Autodesk Inventor part; units mm, degrees
ref_plane "YZ Plane" through (0, 0, 0) normal (1, 0, 0) x (0, 1, 0)
ref_plane "XZ Plane" through (0, 0, 0) normal (0, 1, 0) x (-1, 0, 0)
ref_plane "XY Plane" through (0, 0, 0) normal (0, 0, 1) x (1, 0, 0)
sketch "Sketch1" plane through (0, 0, 0) normal (1, 0, 0) x (0, 1, 0)
  circle A0 centre (0, 0) radius 136.5
  dimension "d0" = 273
extrude "Extrude1" add sketch "Sketch1" along normal blind 432
sketch "Sketch2" plane through (0, 0, 0) normal (0, 0, 1) x (1, 0, 0)
  line L0 (0, 136.5) -> (0, -136.5)
  line L1 (432, 136.5) -> (432, -136.5)
  line L2 (0, 0) -> (432, 0) construction
  circle A0 centre (216, 0) radius 57.15
  dimension "d3" = 114.3
extrude "Extrude2" add sketch "Sketch2" along normal blind 184
sketch "Sketch3" plane through (0, 0, 0) normal (-1, 0, 0) x (0, 0, 1)
  circle A0 centre (0, 0) radius 136.5
  circle A1 centre (0, 0) radius 130.2
  dimension "a" = 216
  dimension "d6" = 260.4
extrude "Extrude3" cut sketch "Sketch3" against normal through all contours A1
sketch "Sketch4" plane through (216, 0, 184) normal (0, 0, 1) x (1, 0, 0)
  circle A0 centre (0, 0) radius 57.15
  circle A1 centre (0, 0) radius 53.55
  dimension "d9" = 107.1
extrude "Extrude4" cut sketch "Sketch4" against normal up to next contours A1
equation "\"d0\" = D1"
equation "\"d1\" = 2 * a"
equation "\"d3\" = D2"
equation "\"d4\" = b"
equation "\"a\" = 216"
equation "\"d6\" = D1 - 2 * s1"
equation "\"d7\" = a"
equation "\"d9\" = D2 - 2 * s2"
equation "\"d10\" = a"
equation "\"D1\" = 273"
equation "\"s1\" = 6.3"
equation "\"D2\" = 114.3"
equation "\"s2\" = 3.6"
equation "\"b\" = 184"
equation "\"Size_Designation\" = 1.2345"
properties part number "DIN 2615-1 Переходный тройник 273 x 6.3 - 114.3 x 3.6 S" material "Сталь"
Could you check a few things on this model? Use its own coordinates, in mm. A direction names the side the tool comes from. Give positions to 0.01 mm unless a question says otherwise; leave off trailing zeros. Order: outer loops, then holes, each group sorted by start corner. A loop starts at its lowest first (then second) coordinate and runs counter-clockwise, first axis right, second up.
1. Thinking about a two-plate mould opening in X: for faces 3 (the cylindrical face through (265.467, -20.51, 151.795)), 4 (the flat face through (432, 121, -50)), 5 (the cylindrical face through (212.976, 5.725, -130.074)), which applies, +X half, -X half, draft (parallel to the pull), parting line (faces both ways), or undercut?
Answers below:
face 3: undercut
face 4: +X half
face 5: draft
2. Which directions (+Z, -Z, +X, -X, +Y, -Y) give clear straight access to the entire face, cutting with the end or side of a thin tool? Please do faces 1 (the flat face through (0, 121, -50)), 2 (the cylindrical face through (170.648, 34.775, 153.559)).
Answers below:
face 1: +Z, -Z, -X, +Y, -Y
face 2: +Z
3. Suppose I cut it at C-C (x = 216). Write out the boundary of the cut face in (y, z), plus the area to 3 significant figures.
Answers below:
outline: (-57.15, 123.96) arc R136.5 ccw (long way) to (57.15, 123.96) - (57.15, 184) - (53.55, 184) - (53.55, 118.68) arc R130.2 cw (long way) to (-53.55, 118.68) - (-53.55, 184) - (-57.15, 184) - close
area: 5,010 mm2
4. Suppose I cut it at A-A (y = 0). Write out the boundary of the cut face in (x, z), plus the area to 3 significant figures.
Answers below:
outline: (0, -136.5) - (432, -136.5) - (432, -130.2) - (0, -130.2) - close; (0, 130.2) - (162.45, 130.2) - (162.45, 184) - (158.85, 184) - (158.85, 136.5) - (0, 136.5) - close; (269.55, 130.2) - (432, 130.2) - (432, 136.5) - (273.15, 136.5) - (273.15, 184) - (269.55, 184) - close
area: 5,110 mm2
5. I need wall thicknesses on L1, parallel to Y at x = 216, z = 168; L2, parallel to X at y = 0, z = 148.5; L3, parallel to Y at x = 354.5, z = 9.5. Which ranges of each line are inside material? Lowest first, please.
Answers below:
L1: y = -57.15 to -53.55, 53.55 to 57.15
L2: x = 158.85 to 162.45, 269.55 to 273.15
L3: y = -136.17 to -129.85, 129.85 to 136.17
6. Suppose I cut it at B-B (z = 0). Write out the boundary of the cut face in (x, y).
Answers below:
outline: (0, -136.5) - (432, -136.5) - (432, -130.2) - (0, -130.2) - close; (0, 130.2) - (432, 130.2) - (432, 136.5) - (0, 136.5) - close
7. Suppose I cut it at D-D (x = 304). Write out the boundary of the cut face in (y, z), plus the area to 3 significant figures.
Answers below:
outline: circle Ø273 at (0, 0); hole circle Ø260.4 at (0, 0)
area: 5,280 mm2
8. For pin 1 (10 mm diameter, centred on x = 92.5, z = -27.5, fed in from -Y); pin 2 (2 mm diameter, centred on x = 143.5, y = 106, fed in from +Z); pin 3 (10 mm diameter, centred on x = 80.5, z = 90, fed in from +Y), each with a flat end and sliding along its axis, tell me the tip position at first contact or that it passes through.
Answers below:
pin 1: stops at y = -134.63
pin 2: stops at z = 87.22
pin 3: stops at y = 106.8
